Autodesk Inventor part; units mm, degrees
ref_plane "YZ Plane" through (0, 0, 0) normal (1, 0, 0) x (0, 1, 0)
ref_plane "XZ Plane" through (0, 0, 0) normal (0, 1, 0) x (-1, 0, 0)
ref_plane "XY Plane" through (0, 0, 0) normal (0, 0, 1) x (1, 0, 0)
sketch "Sketch1" plane through (0, 0, 0) normal (0, 0, 1) x (1, 0, 0)
  line L0 (0, 0) -> (6.25, 0)
  line L1 (6.25, 0) -> (6.25, 8)
  line L2 (6.25, 8) -> (0, 8)
  line L3 (0, 8) -> (0, 0)
  line L4 (6.25, 0) -> (10.25, 0)
  line L5 (10.25, 0) -> (10.25, 8)
  line L6 (10.25, 8) -> (6.25, 8)
  line L7 (6.25, 8) -> (6.25, 0)
  line L8 (0, 0) -> (-4, 0)
  line L9 (-4, 0) -> (-4, 8)
  line L10 (-4, 8) -> (0, 8)
  line L11 (0, 8) -> (0, 0)
  point P0 (6.25, 4)
  point P1 (3.125, 8)
  dimension "d0" = 6.25
  dimension "d1" = 8
  dimension "d3" = 4
extrude "Extrusion1" add sketch "Sketch1" along normal blind 9.15 contours L8 L9 L10 L3 | L1 L6 L5 L4
extrude "Extrusion2" add sketch "Sketch1" against normal blind 4
sketch "Sketch2" plane through (10.25, 0, 9.15) normal (1, 0, 0) x (0, 0, -1)
  line L0 (9.15, 0) -> (9.15, 8)
  line L1 (9.15, 8) -> (0, 8)
  line L2 (0, 0) -> (0, 8)
  line L3 (9.15, 0) -> (0, 0)
  circle A0 centre (4.575, 4) radius 1.6
  line L4 (0, 0) -> (0, 8)
  point P0 (0, 4)
  point P1 (4.575, 8)
  dimension "d8" = 3.2
extrude "Extrusion3" cut sketch "Sketch2" against normal through all contours A0
extrude "Extrusion4" add sketch "Sketch1" along normal blind 4 from surface at 9.15
sketch "Sketch3" plane through (10.25, 0, -4) normal (1, 0, 0) x (0, 0, -1)
  line L0 (-17.15, 17.9016) -> (-17.15, -9.9016)
  line L1 (-17.15, -9.9016) -> (0, 0)
  line L2 (0, 0) -> (0, 8)
  line L3 (0, 8) -> (-17.15, 17.9016)
  line L4 (-17.15, 8) -> (-17.15, 0)
  circle A0 centre (-8.575, 4) radius 1.6
  line L5 (0, 0) -> (-17.15, 0)
  line L6 (-19.475, 19.2439) -> (-19.475, -11.2439)
  line L7 (-17.15, 17.9016) -> (-19.475, 19.2439)
  line L8 (-19.475, -11.2439) -> (-17.15, -9.9016)
  line L9 (-17.15, 0) -> (-19.475, 0)
  point P0 (-4, 0)
  dimension "d13" = 60
  dimension "d20" = 2.325
sketch "Sketch4" plane through (-4, 8, -4) normal (0, 1, 0) x (1, 0, 0)
  line L0 (4, -13.15) -> (10.25, -13.15)
  line L1 (10.25, -4) -> (10.25, -13.15)
  line L2 (4, -4) -> (4, -13.15)
  line L3 (10.25, -4) -> (4, -4)
extrude "Extrusion5" add sketch "Sketch3" against normal up to surface (14.25 mm away) contours L3 L2 L5 L0 | L0 L9 L6 L7
extrude "Extrusion6" cut sketch "Sketch4" along normal through all both and the other way through all
sketch "Sketch5" plane through (10.25, 0, 15.475) normal (1, 0, 0) x (0, 0, -1)
  circle A0 centre (10.9, 4) radius 1.6
  line L0 (19.475, 8) -> (0, 19.2439)
  line L1 (0, 19.2439) -> (0, 0)
  line L2 (19.475, 0) -> (0, 0)
  line L3 (19.475, 8) -> (19.475, 0)
  line L4 (4, 16.9345) -> (4, 0)
  point P0 (15.475, 0)
  dimension "d21" = 4
extrude "Extrusion7" add sketch "Sketch5" along normal blind 10.375 and the other way blind 24.625 contours L4 L2 L1 L0
sketch "Sketch6" plane through (10.25, 0, 11.475) normal (0, 0, -1) x (-1, 0, 0)
  circle A0 centre (-6.6625, 13.2) radius 1.6
  line L0 (-10.375, 0) -> (-10.375, 16.9345)
  line L1 (0, 16.9345) -> (-10.375, 16.9345)
  circle A1 centre (20.9125, 13.2) radius 1.6
  circle A2 centre (20.9125, 4) radius 1.6
  circle A3 centre (-6.6625, 4) radius 1.6
  line L2 (0, 0) -> (-10.375, 0)
  line L3 (24.625, 16.9345) -> (24.625, 0)
  point P0 (10.25, 0)
  dimension "d26" = 3.2
  dimension "d27" = 3.7125
  dimension "d29" = 4
  dimension "d30" = 3.7125
  dimension "d34" = 6
extrude "Extrusion8" cut sketch "Sketch6" against normal through all
fillet "Fillet1" radius 2 4 edges at (10.25, 8.4672, 11.475) (-4, 8.4672, 11.475) (10.25, 4, -4) (-4, 4, -4)
properties part number "TopMotorMount"
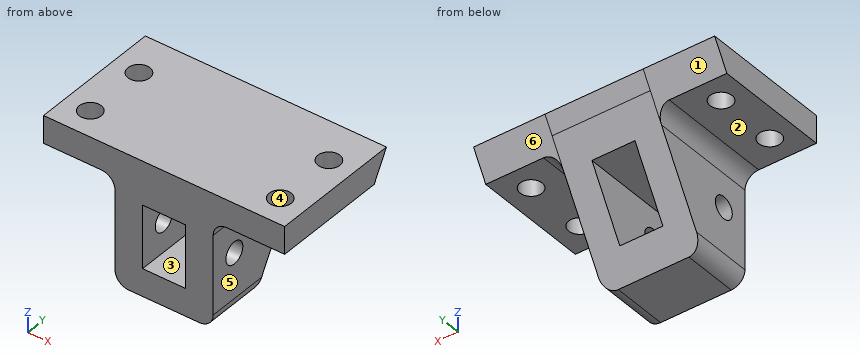
Model file for the job. Use its own axes, mm. Face numbers are marked on the shaded views. A direction names the side the tool comes from. Round coordinates to 2 decimals unless told otherwise and drop trailing zeros. Loops run counter-clockwise (first coordinate to the right, second up) from the corner with the lowest first, then second, coordinate; pieces in that order, holes last.
1. Band-saw the part on B-B, the plane x = 3.5. List the corners of the cut face in (y, z) (3 decimals), and give its area (3 significant figures).
Check values:
outline: (0, -4) - (8, -4) - (10.309, 0) - (0, 0) - close; (0, 9.15) - (15.592, 9.15) - (17.902, 13.15) - (19.244, 15.475) - (0, 15.475) - close
area: 147 mm2
2. Band-saw the part on C-C, the plane y = 6.5. List the corners of the cut face in (x, z) (3 decimals), and give its area (3 significant figures).
Check values:
outline: (-14.375, 11.475) - (-6, 11.475) arc R2 cw to (-4, 9.475) - (-4, -2) arc R2 ccw to (-2, -4) - (8.25, -4) arc R2 ccw to (10.25, -2) - (10.25, 9.475) arc R2 cw to (12.25, 11.475) - (20.625, 11.475) - (20.625, 15.475) - (-14.375, 15.475) - close; hole (0, 0) - (6.25, 0) - (6.25, 9.15) - (0, 9.15) - close
area: 303 mm2
3. Band-saw the part on A-A, the plane y = 4. Count the separate pieces of the cut face and the enclosed holes in it, and give its area (3 significant figures).
Check values:
separate pieces: 4
enclosed holes: 0
area: 252 mm2
4. Drop flat-ended pins along their axis: P1, Ø1, axis at x = -2.5, z = 9, coming from the +Y side; P2, Ø5, axis at y = 4, z = 4.575, coming from the -X side; P3, Ø7.5, axis at y = 5, z = 6, coming from the +X side; P4, Ø5, axis at x = -10.66, y = 4, coming from the +Z side (3 decimals). Give the stop position or say it passes through.
Check values:
P1: stops at y = 15.79
P2: stops at x = -4
P3: stops at x = 10.27
P4: stops at z = 15.475
5. Tool access for the marked faces 1, 2 and 3: list every direction of +Z, -Z, +X, -X, +Y, -Y with a clear straight run to the whole face (end or side of a thin tool).
Check values:
face 1: -Z, +X, -X, +Y
face 2: -Z, -X, +Y, -Y
face 3: +Y, -Y
6. Band-saw the part on D-D, the plane z = 8.5. List the corners of the cut face in (x, y).
Check values:
outline: (-4, 0) - (0, 0) - (0, 15.22) - (-4, 15.22) - close; (6.25, 0) - (10.25, 0) - (10.25, 15.22) - (6.25, 15.22) - close
7. Mould opens along Y. For the marked faces 4, 5 and 6 say: +Y half, -Y half, draft (parallel to the pull), parting line (faces both ways), or undercut.
Check values:
face 4: undercut
face 5: draft
face 6: +Y half
8. Wall check: probe 1 along X at (y, z) = (7.5, 0.75); probe 2 along Z at (x, y) = (4, 5) (3 decimals); probe 3 along Z at (x, y) = (18.5, 16.75) (3 decimals). Give the ranges that are in metal, low to high.
Check values:
probe 1: x = -4 to 0, 6.25 to 10.25
probe 2: z = -4 to 0, 9.15 to 15.475
probe 3: z = 11.475 to 15.475
